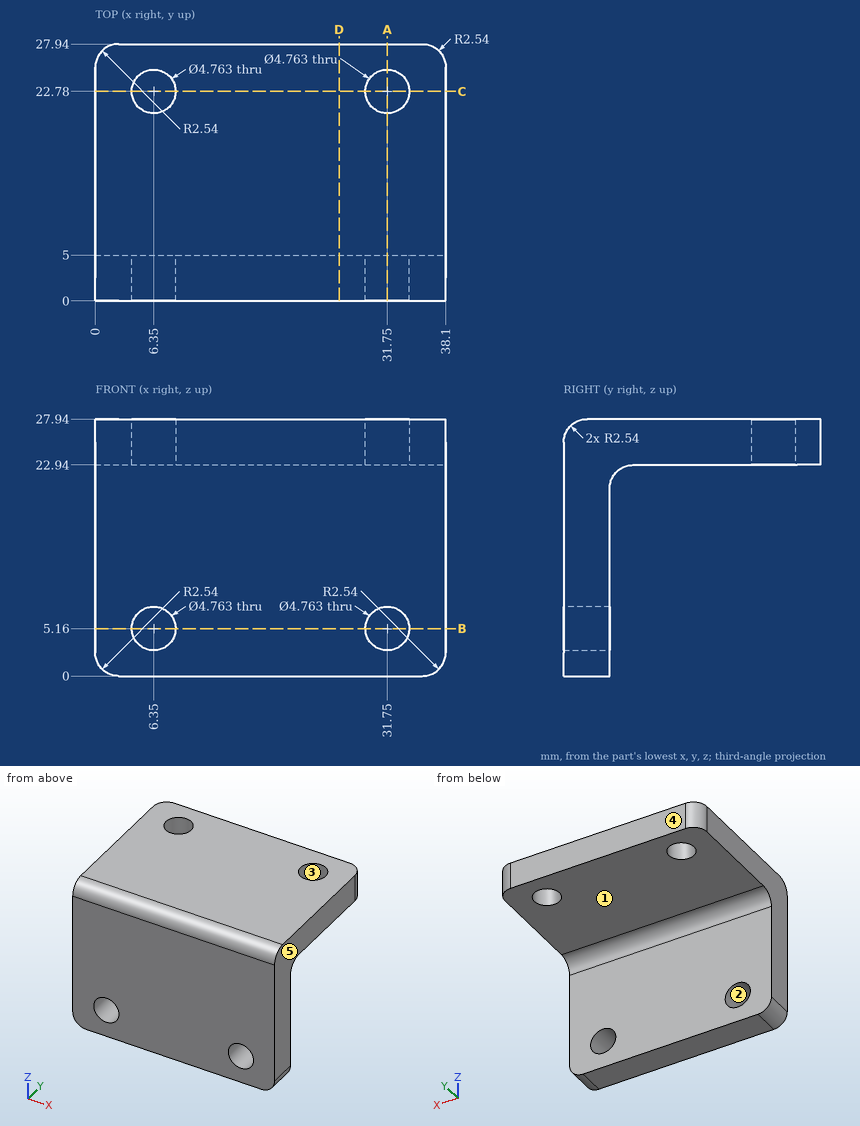
Print and shaded views of the part. All mm, measured from the part's lowest x, y and z. A direction names the side the tool comes from. Give positions to 0.01 mm unless a question says otherwise; leave off trailing zeros. Loops run counter-clockwise (first coordinate to the right, second up) from the corner with the lowest first, then second, coordinate; pieces in that order, holes last. Notation, with made-up numbers: (55.25, 52) -> (81.25, 52) arc R24 cw to (81.25, 83) -> close; hole circle Ø9 at (89, -39). An arc over 180 degrees is marked (long way). Answer in a Markdown table with one row per item.
Item 1: Probe line 1 along X through (y, z) = (2.65, 5.16); line 2 along Y through (x, z) = (6.35, 24.65); line 3 along Z through (x, y) = (12, 24). List the from-to ranges inside material, lowest first. Write a range as [from, to].
Findings below:
| item | result |
|---|---|
| line 1 | x = [0, 3.97], [8.73, 29.37], [34.13, 38.1] |
| line 2 | y = [0, 20.4], [25.16, 27.94] |
| line 3 | z = [22.94, 27.94] |
Item 2: Slice it at B-B on z = 5.16. Write the cut outline in (x, y).
Findings below:
| item | result |
|---|---|
| outline | (0, 0) -> (3.97, 0) -> (3.97, 5) -> (0, 5) -> close; (8.73, 0) -> (29.37, 0) -> (29.37, 5) -> (8.73, 5) -> close; (34.13, 0) -> (38.1, 0) -> (38.1, 5) -> (34.13, 5) -> close |
Item 3: Slice it at C-C on y = 22.78. Write the cut outline in (x, z).
Findings below:
| item | result |
|---|---|
| outline | (0, 22.94) -> (3.97, 22.94) -> (3.97, 27.94) -> (0, 27.94) -> close; (8.73, 22.94) -> (29.37, 22.94) -> (29.37, 27.94) -> (8.73, 27.94) -> close; (34.13, 22.94) -> (38.1, 22.94) -> (38.1, 27.94) -> (34.13, 27.94) -> close |
Item 4: Tool access for the marked faces 1 and 2: list every direction of +Z, -Z, +X, -X, +Y, -Y with a clear straight run to the whole face (end or side of a thin tool).
Findings below:
| item | result |
|---|---|
| face 1 | -Z, +X, -X, +Y |
| face 2 | +Y, -Y |
Item 5: Slice it at A-A on x = 31.75. Write the cut outline in (y, z).
Findings below:
| item | result |
|---|---|
| outline | (0, 0) -> (5, 0) -> (5, 2.78) -> (0, 2.78) -> close; (0, 7.54) -> (5, 7.54) -> (5, 20.4) arc R2.54 cw to (7.54, 22.94) -> (20.4, 22.94) -> (20.4, 27.94) -> (2.54, 27.94) arc R2.54 ccw to (0, 25.4) -> close; (25.16, 22.94) -> (27.94, 22.94) -> (27.94, 27.94) -> (25.16, 27.94) -> close |
Item 6: Mould opens along X. For the marked faces 3, 4 and 5 say: pulls with the +X half, pulls with the -X half, needs draft (parallel to the pull), parting line crosses it, or undercut.
Findings below:
| item | result |
|---|---|
| face 3 | undercut |
| face 4 | needs draft |
| face 5 | pulls with the +X half |
Item 7: Slice it at D-D on x = 26.5. Write the cut outline in (y, z).
Findings below:
| item | result |
|---|---|
| outline | (0, 0) -> (5, 0) -> (5, 20.4) arc R2.54 cw to (7.54, 22.94) -> (27.94, 22.94) -> (27.94, 27.94) -> (2.54, 27.94) arc R2.54 ccw to (0, 25.4) -> close |
Item 8: Flat gauge pins, fed straight in: P1, Ø12, axis at x = 10.5, z = 9, coming from the +Y side; P2, Ø8, axis at x = 17.5, y = 12.5, coming from the -Z side; P3, Ø4.5, axis at x = 6.35, y = 22.78, coming from the -Z side; P4, Ø6, axis at x = 6.35, z = 5.16, coming from the -Y side. Where does each tip first touch, or does it go through?
Findings below:
| item | result |
|---|---|
| P1 | stops at y = 5 |
| P2 | stops at z = 22.94 |
| P3 | passes through |
| P4 | stops at y = 0 |
